Source: CAD feature listing. Evaluate the final solid. Frame: model axes, mm. A direction names the side the tool comes from. Coordinates: 2 decimals unless noted, no trailing zeros. Order: outer loops, then holes, each group sorted by start corner. A loop starts at its lowest first (then second) coordinate and runs counter-clockwise, first axis right, second up.
Solid Edge part; units mm, degrees
sketch "Sketch1" plane through (0, 0, 0) normal (0, 0, 1) x (1, 0, 0)
  circle A0 centre (0, 0) radius 9.398
extrude "Protrusion1" add sketch "Sketch1" along normal blind 5.715
sketch "Sketch2" plane through (0, 0, 0) normal (0, 0, -1) x (1, 0, 0)
  circle A0 centre (0, 0) radius 4.7625
extrude "Protrusion2" add sketch "Sketch2" along normal blind 64.135
sketch "Sketch3" plane through (0, 0, -64.135) normal (0, 0, -1) x (1, 0, 0)
  circle A0 centre (0, 0) radius 4.7622
extrude "Cutout1" cut sketch "Sketch3" against normal blind 25.4 flip side to cut
chamfer "Chamfer_1" distance 0.7144 angle 45 1 edges at (-4.7622, 0, -64.135)
sketch "Sketch4" plane through (0, 0, 5.715) normal (0, 0, 1) x (1, 0, 0)
  line L0 (-1.604, 2.7781) -> (1.604, 2.7781)
  line L1 (3.2079, 0) -> (1.604, 2.7781)
  line L2 (1.604, -2.7781) -> (3.2079, 0)
  line L3 (-1.604, -2.7781) -> (1.604, -2.7781)
  line L4 (-3.2079, 0) -> (-1.604, -2.7781)
  line L5 (-1.604, 2.7781) -> (-3.2079, 0)
extrude "Cutout2" cut sketch "Sketch4" against normal blind 3.81
sketch "Sketch5" plane through (0, 0, 0) normal (0, -1, 0) x (1, 0, 0)
  line L0 (9.398, 5.715) -> (4.43, 0)
  line L1 (4.43, 0) -> (9.398, 0)
  line L2 (9.398, 0) -> (9.398, 5.715)
revolve "RevolvedCutout1" cut sketch "Sketch5" angle 360 about axis through (0, 0, 14.0017) along (0, 0, -1)
properties part number "185727" material "Stainless Steel, 304"
1. Material intervals for line 1 along X through (y, z) = (2.5, -41); line 2 along Z through (x, y) = (-1.5, -0.5) (3 decimals); line 3 along Y through (x, z) = (-1.5, -10), sorted ascending.
2. Draft query along X for faces 1 (the flat face through (-2.2, 2.2, 5.715)), 2 (the flat face through (2.4, 1.4, 3.8)), 3 (the cylindrical face through (-3.779, 2.898, -51.251)). Return one class per face: +X half, -X half, draft (parallel to the pull), parting line (faces both ways), or undercut.
3. Contact query for flat-ended pins moving along their axis: P1, Ø1.5, axis at x = 4.5, z = -47.5, coming from the +Y side; P2, Ø1.7, axis at x = -0.5, y = 1, coming from the +Z side (3 decimals); P3, Ø3, axis at x = -2, z = -51, coming from the -Y side; P4, Ø4, axis at x = 7.5, z = -37.5, coming from the -Y side. Output: stop coordinate, or through.
4. Section query B-B, the plane z = -56.5. Output: boundary loops of the cut face in (x, y), plus the area to 3 significant figures.
5. Access query for faces 4 (the flat face through (-2.4, -1.4, 3.8)), 5 (the cylindrical face through (-3.78, -2.9, -19.1)), 6 (the flat face through (0, 0, -64.135)). Directions: +Z, -Z, +X, -X, +Y, -Y. A direction counts if a zero-diameter tool reaches every point of the face in a straight line with its end or side. Return the directions, or none.
6. Section query C-C, the plane z = -11. Output: boundary loops of the cut face in (x, y) (1 decimal).
Answer key:
1. line 1: x = -4.05 to 4.05
1. line 2: z = -64.135 to 1.905
1. line 3: y = -4.52 to 4.52
2. face 1: draft
2. face 2: undercut
2. face 3: parting line
3. P1: stops at y = 2.94
3. P2: stops at z = 1.905
3. P3: stops at y = -4.74
3. P4: passes through
4. outline: circle Ø9.52 at (0, 0)
4. area: 71.2 mm2
5. face 4: +Z
5. face 5: -Z
5. face 6: -Z, +X, -X, +Y, -Y
6. outline: circle Ø9.5 at (0, 0)
